```python
from build123d import *

# Parameters (mm, degrees)
F1_DEPTH = 65
F2_R     = 2
F3_R     = 1


with BuildPart() as f1:
    # F0 (on Top) → F1 (new body)
    with BuildSketch(Plane.XY):
        Polygon((0, 15), (0, 0), (1, 0), (1, 11), (4.2, 11), (4.2, 8), (3.1, 8), (3.1, 7), (4.2, 7), (8.2, 7), (8.2, 15), align=None)
    extrude(amount=F1_DEPTH)

    # F2
    f2_edges = [f1.edges().sort_by_distance(p)[0] for p in [
        (8.2, 15, 32.5),
        (0, 15, 32.5),
    ]]
    fillet(f2_edges, radius=F2_R)

    # F3
    f3_edges = [f1.edges().sort_by_distance(p)[0] for p in [
        (8.2, 7, 32.5),
    ]]
    fillet(f3_edges, radius=F3_R)


solid = f1.part
```
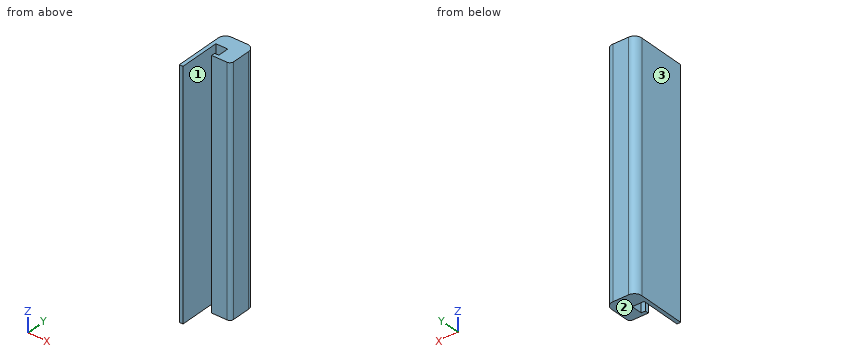
Could you check a few things on this model? Use its own coordinates, in mm. Face numbers are marked on the shaded views. Give positions to 0.01 mm unless a question says otherwise; leave off trailing zeros. Order: outer loops, then holes, each group sorted by start corner. A loop starts at its lowest first (then second) coordinate and runs counter-clockwise, first axis right, second up.
Q1. I'm going to push flat-ended pins straight in: P1, Ø1, axis at y = 7.5, z = 38.5, coming from the +X side; P2, Ø1.5, axis at x = 6.5, z = 15.5, coming from the -Y side; P3, Ø2, axis at y = 2, z = 56.5, coming from the +X side. Where does each tip first touch, or does it pass through?
Q2. Suppose I cut it at C-C, the plane x = 4.75. Write out the boundary of the cut face in (y, z).
Q3. Suppose I cut it at B-B, the plane y = 5.75. Write out the boundary of the cut face in (x, z), and give its area (3 significant figures).
Q4. We'd pull the mould along X, two halves only. Please class the marked faces 1, 2 and 3: +X half, -X half, draft (parallel to the pull), parting line (faces both ways), or undercut.
Q5. If I drill on line 1 along X through (y, z) = (9, 10); line 2 along Y through (x, z) = (3, 12); line 3 along Y through (x, z) = (5.5, 48.5), over which ranges is the centre line in solid material (lowest first)?
Q6. Suppose I cut it at A-A, the plane z = 9. Write out the boundary of the cut face in (x, y), and give its area (3 significant figures).
Solution:
1. P1: stops at x = 8.2
1. P2: stops at y = 7
1. P3: stops at x = 1
2. outline: (7, 0) - (15, 0) - (15, 65) - (7, 65) - close
3. outline: (0, 0) - (1, 0) - (1, 65) - (0, 65) - close
3. area: 65.0 mm2
4. face 1: undercut
4. face 2: draft
4. face 3: -X half
5. line 1: x = 0 to 1, 4.2 to 8.2
5. line 2: y = 11 to 15
5. line 3: y = 7 to 15
6. outline: (0, 0) - (1, 0) - (1, 11) - (4.2, 11) - (4.2, 8) - (3.1, 8) - (3.1, 7) - (7.2, 7) arc R1 ccw to (8.2, 8) - (8.2, 13) arc R2 ccw to (6.2, 15) - (2, 15) arc R2 ccw to (0, 13) - close
6. area: 59.0 mm2
